from build123d import *

# Parameters (mm, degrees)
F0_W     = 191.008
F0_H     = 50.8
F1_DEPTH = 21.336
F2_W     = 36.322
F2_H     = 47.625
F3_DEPTH = 191.009


with BuildPart() as f1:
    # F0 (on Front) → F1 (new body, symmetric)
    with BuildSketch(Plane.XZ):
        with Locations((95.504, 25.4)):
            Rectangle(F0_W, F0_H)
    extrude(amount=F1_DEPTH, both=True)

    # F2 (on Right) → F3 (cut, through all)
    with BuildSketch(Plane.YZ):
        with Locations((0, 26.9875)):
            Rectangle(F2_W, F2_H)
    extrude(amount=F3_DEPTH, mode=Mode.SUBTRACT)


solid = f1.part
Could you check a few things on this model? Use its own coordinates, in mm. A direction names the side the tool comes from. Give positions to 0.01 mm unless a question says otherwise; leave off trailing zeros. Order: outer loops, then holes, each group sorted by start corner. A loop starts at its lowest first (then second) coordinate and runs counter-clockwise, first axis right, second up.
1. Suppose I cut it at A-A (z = 26.5). Write out the boundary of the cut face in (x, y).
Answers below:
outline: (0, -21.34) - (191.01, -21.34) - (191.01, -18.16) - (0, -18.16) - close; (0, 18.16) - (191.01, 18.16) - (191.01, 21.34) - (0, 21.34) - close
2. I need wall thicknesses on L1, parallel to Y at x = 70, z = 17.5; L2, parallel to Z at x = 33, y = 13.5 (3 decimals). Which ranges of each line are inside material? Lowest first, please.
Answers below:
L1: y = -21.34 to -18.16, 18.16 to 21.34
L2: z = 0 to 3.175
3. Thinking about a two-plate mould opening in Y: for faces 1 (the flat face through (94, 18.161, 27)), 2 (the flat face through (191.008, 1, 3)), 3 (the flat face through (94, 0, 3.175)), 4 (the flat face through (94, 21.336, 26)), which applies, +Y half, -Y half, draft (parallel to the pull), parting line (faces both ways), or undercut?
Answers below:
face 1: undercut
face 2: draft
face 3: undercut
face 4: +Y half
4. Suppose I cut it at C-C (y = -1). Write out the boundary of the cut face in (x, z) (3 decimals), plus the area to 3 significant figures.
Answers below:
outline: (0, 0) - (191.008, 0) - (191.008, 3.175) - (0, 3.175) - close
area: 606 mm2
5. Suppose I cut it at B-B (x = 76). Write out the boundary of the cut face in (y, z) (3 decimals).
Answers below:
outline: (-21.336, 0) - (21.336, 0) - (21.336, 50.8) - (18.161, 50.8) - (18.161, 3.175) - (-18.161, 3.175) - (-18.161, 50.8) - (-21.336, 50.8) - close
6. Which directions (+Z, -Z, +X, -X, +Y, -Y) give clear straight access to the entire face, cutting with the end or side of a thin tool? Please do faces 5 (the flat face through (94, -18.161, 27)), 6 (the flat face through (94, -21.336, 26)).
Answers below:
face 5: +Z, +X, -X
face 6: +Z, -Z, +X, -X, -Y
